```python
from build123d import *

# Parameters (mm, degrees)
ESQUISSE1_W             = 130
ESQUISSE1_H             = 65
ESQUISSE1_R             = 1.3
BOSS_EXTRU_1_DEPTH      = 7.8
ESQUISSE2_W             = 130
ESQUISSE2_H             = 12.5
ESQUISSE2_H_2           = 22
ENL_V_MAT_EXTRU_1_DEPTH = 0.5
D_GAGEMENT_M3_D         = 3.4
D_GAGEMENT_M3_DEPTH     = 6.978536948
D_GAGEMENT_M3_TIP       = 1.021463052


with BuildPart() as part:
    # Esquisse1 → Boss.-Extru.1 (new body)
    with BuildSketch(Plane.XY):
        with Locations((65, 32.5)):
            Rectangle(ESQUISSE1_W, ESQUISSE1_H)
        with Locations((113, 5)):
            Circle(ESQUISSE1_R, mode=Mode.SUBTRACT)
        with Locations((89, 5)):
            Circle(ESQUISSE1_R, mode=Mode.SUBTRACT)
        with Locations((65, 5)):
            Circle(ESQUISSE1_R, mode=Mode.SUBTRACT)
        with Locations((41, 5)):
            Circle(ESQUISSE1_R, mode=Mode.SUBTRACT)
        with Locations((17, 5)):
            Circle(ESQUISSE1_R, mode=Mode.SUBTRACT)
        with Locations((113, 60)):
            Circle(ESQUISSE1_R, mode=Mode.SUBTRACT)
        with Locations((89, 60)):
            Circle(ESQUISSE1_R, mode=Mode.SUBTRACT)
        with Locations((65, 60)):
            Circle(ESQUISSE1_R, mode=Mode.SUBTRACT)
        with Locations((41, 60)):
            Circle(ESQUISSE1_R, mode=Mode.SUBTRACT)
        with Locations((17, 60)):
            Circle(ESQUISSE1_R, mode=Mode.SUBTRACT)
    extrude(amount=BOSS_EXTRU_1_DEPTH)

    # Esquisse2 → Enlèv. mat.-Extru.1 (cut)
    with BuildSketch(Plane(origin=(0, 0, 0), x_dir=(-1, 0, 0), z_dir=(0, 0, -1))):
        with Locations((-65, 58.75)):
            Rectangle(ESQUISSE2_W, ESQUISSE2_H)
        with Locations((-65, 6.25)):
            Rectangle(ESQUISSE2_W, ESQUISSE2_H)
        with Locations((-65, 32.5)):
            Rectangle(ESQUISSE2_W, ESQUISSE2_H_2)
    extrude(amount=-ENL_V_MAT_EXTRU_1_DEPTH, mode=Mode.SUBTRACT)

    # Dégagement M3
    with Locations(Plane.XY.offset(7.8)):
        with Locations((17, 60), (41, 60), (65, 60), (89, 60), (113, 60), (113, 5), (89, 5), (65, 5), (41, 5), (17, 5)):
            Hole(D_GAGEMENT_M3_D / 2, depth=D_GAGEMENT_M3_DEPTH)
            with Locations((0, 0, -(D_GAGEMENT_M3_DEPTH + D_GAGEMENT_M3_TIP / 2))):  # 118° drill point
                Cone(0, D_GAGEMENT_M3_D / 2, D_GAGEMENT_M3_TIP, mode=Mode.SUBTRACT)


solid = part.part
```
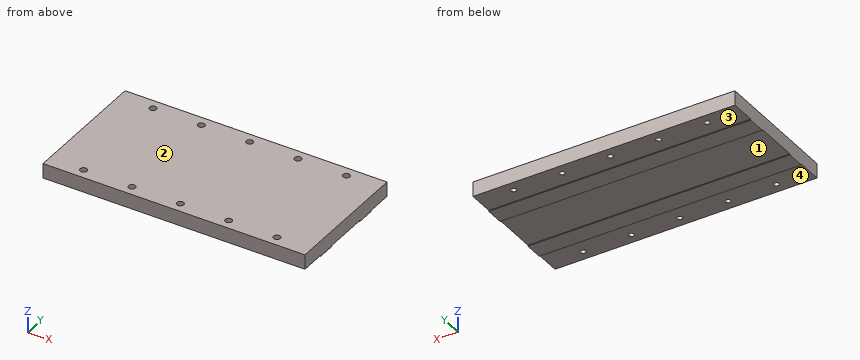
Geometry check sheet. Reference: the model listing, model coordinates, mm. Face numbers are marked on the shaded views. A direction names the side the tool comes from. Give positions to 0.01 mm unless a question says otherwise; leave off trailing zeros. Loops run counter-clockwise (first coordinate to the right, second up) from the corner with the lowest first, then second, coordinate; pieces in that order, holes last. Notation, with made-up numbers: M -20.5,-15.75 L 27.5,-15.75 A32 ccw 27.5,19.25 Z; hole C -27.5,86 d4. An arc over 180 degrees is marked long. Write item = value, one per line. Start each with the question number.
1. Draft check along Y on the marked faces 1 and 2. Enter one of: +Y half, -Y half, draft (parallel to the pull), parting line (faces both ways), or undercut.
2. Tool access check on the marked faces 3 and 4. Record the directions out of +Z, -Z, +X, -X, +Y, -Y that give a thin tool (end or side, any length) a straight path to the whole face; none if there is none.
3. Section check B-B, the plane y = 9.5. Enter the section's corners in (x, z), plus the area to 3 significant figures.
4. Section check A-A, the plane x = 113. Enter the section's corners in (y, z).
5. Thickness scan on probe 1 along Y at (x, z) = (17, 5.5); probe 2 along X at (y, z) = (5, 3.5); probe 3 along X at (y, z) = (60, 0.55). Record the ranges inside material, lowest first.
6. Go/stop test with flat-tipped pins: P1, Ø10, axis at x = 35.5, y = 3.5, coming from the -Z side; P2, Ø2.5, axis at x = 41, y = 5, coming from the +Z side; P3, Ø0.6, axis at x = 88, z = 0, coming from the +Y side. Record where each tip stops, or that it passes through.
Values follow:
q1.face_1 = undercut
q1.face_2 = draft
q2.face_3 = -Z, +X, -X, +Y
q2.face_4 = -Z, +X, -X, -Y
q3.outline = M 0,0.5 L 130,0.5 L 130,7.8 L 0,7.8 Z
q3.area = 949 mm^2
q4.outline = M 0,0.5 L 3.7,0.5 L 3.7,0.58 L 3.3,0.82 L 3.3,7.8 L 0,7.8 Z; M 6.3,0.5 L 12.5,0.5 L 12.5,0 L 21.5,0 L 21.5,0.5 L 43.5,0.5 L 43.5,0 L 52.5,0 L 52.5,0.5 L 58.7,0.5 L 58.7,0.58 L 58.3,0.82 L 58.3,7.8 L 6.7,7.8 L 6.7,0.82 L 6.3,0.58 Z; M 61.3,0.5 L 65,0.5 L 65,7.8 L 61.7,7.8 L 61.7,0.82 L 61.3,0.58 Z
q5.probe_1 = 0 to 3.3, 6.7 to 58.3, 61.7 to 65
q5.probe_2 = 0 to 15.3, 18.7 to 39.3, 42.7 to 63.3, 66.7 to 87.3, 90.7 to 111.3, 114.7 to 130
q5.probe_3 = 0 to 15.7, 18.3 to 39.7, 42.3 to 63.7, 66.3 to 87.7, 90.3 to 111.7, 114.3 to 130
q6.P1 = 0.5
q6.P2 = through
q6.P3 = 52.5
